For this review, take the finished solid that the model builds, in its own axes (mm). Give positions to 0.01 mm unless a question says otherwise; leave off trailing zeros. Loops run counter-clockwise (first coordinate to the right, second up) from the corner with the lowest first, then second, coordinate; pieces in that order, holes last. Notation, with made-up numbers: (-38, -6.5) - (-24, -6.5) arc R17 ccw to (-24, 22.5) - close; hole circle Ø4 at (-20, -6). An arc over 180 degrees is marked (long way). Answer in a Markdown table with one row per item.
```python
from build123d import *
from OCP.BRepAlgoAPI import BRepAlgoAPI_Cut
from OCP.TopTools import TopTools_ListOfShape

# Parameters (mm, degrees)
SKIZZE2_R                       = 8.25
SKIZZE2_R_2                     = 0.8
AUFSATZ_LINEAR_AUSTRAGEN1_DEPTH = 4


with BuildPart() as part:
    # Skizze2 → Aufsatz-Linear austragen1 (new body)
    with BuildSketch(Plane.XY):
        with Locations((-1.64e-06, -6.336e-06)):
            Circle(SKIZZE2_R)
        with Locations((6.000570744, 0.000379921)):
            Circle(SKIZZE2_R_2, mode=Mode.SUBTRACT)
        with Locations((0.000570744, 6.000379921)):
            Circle(SKIZZE2_R_2, mode=Mode.SUBTRACT)
        with Locations((-5.999429256, 0.000379921)):
            Circle(SKIZZE2_R_2, mode=Mode.SUBTRACT)
        with Locations((0.000570744, -5.999620079)):
            Circle(SKIZZE2_R_2, mode=Mode.SUBTRACT)
    extrude(amount=AUFSATZ_LINEAR_AUSTRAGEN1_DEPTH)


with BuildPart() as schnitt_rotation4_tool:
    # Skizze5 → Schnitt-Rotation4 (revolve)
    with BuildSketch(Plane(origin=(0, 0, 0), x_dir=(0, 0, -1), z_dir=(1, 0, 0))):
        with BuildLine():
            Line((-3.25, 8.249993664), (-0.75, 8.249993664))
            ThreePointArc((-0.75, 8.249993664), (-2, 7.480469675), (-3.25, 8.249993664))
        make_face()
    revolve(axis=Axis((0, 0, 2), (0, 0, 1)))


with BuildPart() as part_1:
    add(part.part)

    # Schnitt-Rotation4: cut by schnitt_rotation4_tool, with a tolerance
    schnitt_rotation4_stock = TopTools_ListOfShape()
    schnitt_rotation4_stock.Append(part_1.part.wrapped)
    schnitt_rotation4_tools = TopTools_ListOfShape()
    schnitt_rotation4_tools.Append(schnitt_rotation4_tool.part.wrapped)
    schnitt_rotation4_cut = BRepAlgoAPI_Cut()
    schnitt_rotation4_cut.SetArguments(schnitt_rotation4_stock)
    schnitt_rotation4_cut.SetTools(schnitt_rotation4_tools)
    schnitt_rotation4_cut.SetFuzzyValue(0.00001)
    schnitt_rotation4_cut.Build()
    add(Compound.cast(schnitt_rotation4_cut.Shape()).solids(), mode=Mode.REPLACE)


solid = part_1.part
```
1. Wall thickness on line 1 (Y direction, x = 0.5, z = 0.2); line 2 (Y direction, x = -0.25, z = 1.9); line 3 (Z direction, x = 5.5, y = -6): over which ranges is each line inside the solid? List them lowest first. Write a range as [from, to].
Values:
| item | result |
|---|---|
| line 1 | y = [-8.23, -6.62], [-5.37, 5.38], [6.63, 8.23] |
| line 2 | y = [-7.48, -6.76], [-5.24, 5.24], [6.76, 7.48] |
| line 3 | z = [0, 0.81], [3.19, 4] |
2. Clearance check with flat-ended pins moving along their axes: pin 1 (2 mm diameter, centred on x = 4.5, y = 4.5, fed in from -Z); pin 2 (1.4 mm diameter, centred on x = 0, y = -6, fed in from +Z). State where each tip first meets the part, or that it passes through.
Values:
| item | result |
|---|---|
| pin 1 | stops at z = 0 |
| pin 2 | passes through |
3. Mouldability with a two-part tool opening along X and no side actions: class faces 1 (the face through (0, 0, 0)), 2 (the face through (-5.236, 0.241, 1.972)), 3 (the face through (7.87, 2.48, 0.37)) as released by +X, released by -X, zero draft, split by the parting line, or undercut.
Values:
| item | result |
|---|---|
| face 1 | zero draft |
| face 2 | undercut |
| face 3 | split by the parting line |
4. We need section A-A, the plane z = 1.7. Give the boundary of the cut face in (x, y).
Values:
| item | result |
|---|---|
| outline | circle Ø15.03 at (0, 0); hole circle Ø1.6 at (-6, 0); hole circle Ø1.6 at (0, -6); hole circle Ø1.6 at (0, 6); hole circle Ø1.6 at (6, 0) |
5. We need section B-B, the plane z = 3.6. Give the boundary of the cut face in (x, y), and give its area (3 significant figures).
Values:
| item | result |
|---|---|
| outline | circle Ø16.5 at (0, 0); hole circle Ø1.6 at (-6, 0); hole circle Ø1.6 at (0, -6); hole circle Ø1.6 at (0, 6); hole circle Ø1.6 at (6, 0) |
| area | 206 mm^2 |
